from build123d import *

# Parameters (mm, degrees)
SKETCH1_R           = 2.38
BOSS_EXTRUDE1_DEPTH = 12.64
CHAMFER1_SIZE       = 4.2291
CHAMFER1_SIZE2      = 2.94


with BuildPart() as part:
    # Sketch1 → Boss-Extrude1 (new body)
    with BuildSketch(Plane(origin=(0, 0, 0), x_dir=(1, 0, 0), z_dir=(0, 1, 0))):
        with BuildLine():
            Line((279.847634913, -120.65), (-279.847634913, -120.65))
            ThreePointArc((-279.847634913, -120.65), (-326.268482654, -109.291064504), (-362.199527238, -77.781057273))
            ThreePointArc((-362.199527238, -77.781057273), (-388.816521313, -54.439078616), (-423.204150273, -46.024608002))
            Line((-423.204150273, -46.024608002), (-476.469252285, -46.024608002))
            ThreePointArc((-476.469252285, -46.024608002), (-509.344325494, -32.599702877), (-523.424733457, 0))
            ThreePointArc((-523.424733457, 0), (-509.344325494, 32.599702877), (-476.469252285, 46.024608002))
            Line((-476.469252285, 46.024608002), (-423.204150273, 46.024608002))
            ThreePointArc((-423.204150273, 46.024608002), (-388.816521313, 54.439078616), (-362.199527238, 77.781057273))
            ThreePointArc((-362.199527238, 77.781057273), (-326.268482654, 109.291064504), (-279.847634913, 120.65))
            Line((-279.847634913, 120.65), (279.847634913, 120.65))
            ThreePointArc((279.847634913, 120.65), (326.268482654, 109.291064504), (362.199527238, 77.781057273))
            ThreePointArc((362.199527238, 77.781057273), (388.816521313, 54.439078616), (423.204150273, 46.024608002))
            Line((423.204150273, 46.024608002), (476.469252285, 46.024608002))
            ThreePointArc((476.469252285, 46.024608002), (509.344325494, 32.599702877), (523.424733457, 0))
            ThreePointArc((523.424733457, 0), (509.344325494, -32.599702877), (476.469252285, -46.024608002))
            Line((476.469252285, -46.024608002), (423.204150273, -46.024608002))
            ThreePointArc((423.204150273, -46.024608002), (388.816521313, -54.439078616), (362.199527238, -77.781057273))
            ThreePointArc((362.199527238, -77.781057273), (326.268482654, -109.291064504), (279.847634913, -120.65))
        make_face()
        with Locations(Location((-404.164718127, 20.6375, 0), (0, 0, 90))):
            Circle(SKETCH1_R, mode=Mode.SUBTRACT)
        with Locations(Location((-462.266329753, 20.6375, 0), (0, 0, 90))):
            Circle(SKETCH1_R, mode=Mode.SUBTRACT)
        with Locations(Location((-404.164718127, -20.6375, 0), (0, 0, 90))):
            Circle(SKETCH1_R, mode=Mode.SUBTRACT)
        with Locations(Location((-462.266329753, -20.6375, 0), (0, 0, 90))):
            Circle(SKETCH1_R, mode=Mode.SUBTRACT)
        with Locations(Location((462.266329753, -20.6375, 0), (0, 0, 90))):
            Circle(SKETCH1_R, mode=Mode.SUBTRACT)
        with Locations(Location((404.164718127, -20.6375, 0), (0, 0, 90))):
            Circle(SKETCH1_R, mode=Mode.SUBTRACT)
        with Locations(Location((462.266329753, 20.6375, 0), (0, 0, 90))):
            Circle(SKETCH1_R, mode=Mode.SUBTRACT)
        with Locations(Location((404.164718127, 20.6375, 0), (0, 0, 90))):
            Circle(SKETCH1_R, mode=Mode.SUBTRACT)
    extrude(amount=BOSS_EXTRUDE1_DEPTH)

    # Chamfer1
    chamfer1_edges = [part.edges().sort_by_distance(p)[0] for p in [
        (-462.266329753, 12.64, -18.2575),
        (-404.164718127, 12.64, 23.0175),
        (-462.266329753, 12.64, 23.0175),
        (-404.164718127, 12.64, -18.2575),
        (462.266329753, 12.64, 23.0175),
        (404.164718127, 12.64, 23.0175),
        (462.266329753, 12.64, -18.2575),
        (404.164718127, 12.64, -18.2575),
    ]]
    chamfer1_side = [part.faces().sort_by_distance(p)[0] for p in [
        (0, 12.64, 0),
    ]]
    chamfer(chamfer1_edges, length=CHAMFER1_SIZE, length2=CHAMFER1_SIZE2, reference=chamfer1_side[0])


solid = part.part
Verification items for the finished model (mm, model axes). Give positions to 0.01 mm unless a question says otherwise; leave off trailing zeros. Write each loop counter-clockwise with the first axis right and the second up, starting at its lowest first coordinate (ties: lowest second). Pieces come first, ordered by that corner, then holes. Notation, with made-up numbers: M -12,-28 L -6,-28 A24 cw -6,-9 Z; hole C 65.25,53.25 d1. An arc over 180 degrees is marked long. Write item = value, one per line.
(1) Sectioned sample at A-A (x = 438). Record the cut outline in (y, z), then the cut area to 3 significant figures.
Found:
outline = M 0,-46.02 L 12.64,-46.02 L 12.64,46.02 L 0,46.02 Z
area = 1,160 mm2
(2) Material ranges on line 1 (Z direction, x = 471.5, y = 1.5); line 2 (X direction, y = 3.5, z = -96.5); line 3 (Z direction, x = -377.5, y = 5.5), recorded low to high.
Found:
line_1 = -46.02 to 46.02
line_2 = -345.21 to 345.21
line_3 = -61.7 to 61.7
(3) Go/stop test with flat-tipped pins: pin 1 Ø4.5 at (x, z) = (-404.16, -20.64) entering from +Y; pin 2 Ø4 at (x, y) = (458, 9.5) entering from -Z; pin 3 Ø1.5 at (x, y) = (376, 6) entering from -Z; pin 4 Ø1.5 at (y, z) = (11, 91.5) entering from +X. Record where each tip stops, or that it passes through.
Found:
pin_1 = through
pin_2 = -46.02
pin_3 = -63.52
pin_4 = 351.39
(4) Sectioned sample at B-B (y = 3.5). Give the number of separate pieces and of enclosed holes in the cut face, then the cut area to 3 significant figures.
Found:
separate_pieces = 1
enclosed_holes = 8
area = 201,000 mm2
(5) Sectioned sample at C-C (z = -55). Record the cut outline in (x, y).
Found:
outline = M -387.76,0 L 387.76,0 L 387.76,12.64 L -387.76,12.64 Z
